Check sheet for the modelled part. Datum: model origin and axes. Units: mm. Face numbers are marked on the shaded views. A direction names the side the tool comes from. Give positions to 0.01 mm unless a question says otherwise; leave off trailing zeros. Write each loop counter-clockwise with the first axis right and the second up, starting at its lowest first coordinate (ties: lowest second). Pieces come first, ordered by that corner, then holes. Notation, with made-up numbers: M 25.5,-11.5 L 82.5,-11.5 A23 ccw 82.5,-0.5 Z; hole C 62,76 d11. An arc over 180 degrees is marked long. Use CSV: the item, a comma, the result in double quotes. Start each with the question number.
1. Cross-section at D-D, the plane y = -23.5. Enter the section's corners in (x, z).
2. Cross-section at C-C, the plane z = 43. Enter the section's corners in (x, y), and give its area (3 significant figures).
3. Depth check by flat-ended pin: P1, Ø1.4, axis at x = -41, y = -39.5, coming from the +Z side; P2, Ø1.5, axis at y = -21, z = 117, coming from the +X side; P3, Ø11, axis at x = -15.5, y = -47, coming from the -Z side; P4, Ø5, axis at x = -32, z = 81, coming from the +Y side. Enter the tip coordinate at first touch or a pass-through.
4. Scan lines: line 1 (Z direction, x = -58, y = -8.5); line 2 (X direction, y = -19, z = 56.5); line 3 (Y direction, x = -10.5, z = 86.5). Record each from-to range of solid material in increasing order.
5. Access from +Z, -Z, +X, -X, +Y, -Y to the whole of each face (thin tool, end or side, straight path). Record for the marked faces 4 and 5.
6. Cross-section at B-B, the plane x = -40. Enter the section's corners in (y, z), and give its area (3 significant figures).
7. Cross-section at A-A, the plane y = -30. Enter the section's corners in (x, z), and give its area (3 significant figures).
8. Mould release check, pull along Z, two halves, no side actions. Record for the marked faces 1, 2 and 3: +Z half, -Z half, draft (parallel to the pull), parting line (faces both ways), or undercut.
from build123d import *

# Parameters (mm, degrees)
F0_W      = 80
F0_H      = 120
F1_DEPTH  = 40
F2_T      = -1.8
F0_H_2    = 10
F3_DEPTH  = 40
F5_DEPTH  = 40
F8_DEPTH  = 5
F9_DEPTH  = 6
F10_DEPTH = 10
F12_DEPTH = 5


with BuildPart() as f1:
    # F0 (on Front) → F1 (new body)
    with BuildSketch(Plane.XZ):
        with Locations((-40, 60)):
            Rectangle(F0_W, F0_H)
    extrude(amount=F1_DEPTH)

    # F2
    f2_openings = [f1.faces().sort_by_distance(p)[0] for p in [
        (-40, 0, 60),
    ]]
    offset(amount=F2_T, openings=f2_openings)

    # F0 (on Front) → F3 (join)
    with BuildSketch(Plane.XZ):
        with Locations((-40, 125)):
            Rectangle(F0_W, F0_H_2)
    extrude(amount=F3_DEPTH)

    # F4 (on face) → F5 (cut)
    with BuildSketch(Plane.XZ):
        Polygon((-42.5, 45), (-40, 45), (-37.5, 45), (-37.5, 75), (-42.5, 75), align=None)
    extrude(amount=F5_DEPTH, mode=Mode.SUBTRACT)

    # F7 (on offset) → F8 (join)
    with BuildSketch(Plane.XY.offset(130)):
        with BuildLine():
            ThreePointArc((-50, 0), (-40, -10), (-30, 0))
            Line((-30, 0), (-40, 0))
            Line((-40, 0), (-50, 0))
        make_face()
    extrude(amount=F8_DEPTH)

    # F7 (on offset) → F9 (cut)
    with BuildSketch(Plane.XY.offset(130)):
        with BuildLine():
            ThreePointArc((-12, -20), (-14.343146, -14.343146), (-20, -12))
            ThreePointArc((-20, -12), (-28, -20), (-20, -28))
            ThreePointArc((-20, -28), (-14.343146, -25.656854), (-12, -20))
        make_face()
        with BuildLine():
            ThreePointArc((-52, -20), (-54.343146, -14.343146), (-60, -12))
            ThreePointArc((-60, -12), (-68, -20), (-60, -28))
            ThreePointArc((-60, -28), (-54.343146, -25.656854), (-52, -20))
        make_face()
    extrude(amount=-F9_DEPTH, mode=Mode.SUBTRACT)

    # F7 (on offset) → F10 (join)
    with BuildSketch(Plane.XY.offset(130)):
        with BuildLine():
            ThreePointArc((-50, -40), (-52.928932, -32.928932), (-60, -30))
            ThreePointArc((-60, -30), (-67.071068, -47.071068), (-50, -40))
        make_face()
        with BuildLine():
            ThreePointArc((-10, -40), (-12.928932, -32.928932), (-20, -30))
            ThreePointArc((-20, -30), (-27.071068, -47.071068), (-10, -40))
        make_face()
    extrude(amount=-F10_DEPTH)

    # F11 (on offset) → F12 (cut)
    with BuildSketch(Plane.XY.offset(130)):
        with BuildLine():
            ThreePointArc((-70, -40), (-60, -50), (-50, -40))
            Line((-50, -40), (-60, -40))
            Line((-60, -40), (-70, -40))
        make_face()
        with BuildLine():
            ThreePointArc((-30, -40), (-20, -50), (-10, -40))
            Line((-10, -40), (-20, -40))
            Line((-20, -40), (-30, -40))
        make_face()
    extrude(amount=-F12_DEPTH, mode=Mode.SUBTRACT)


solid = f1.part
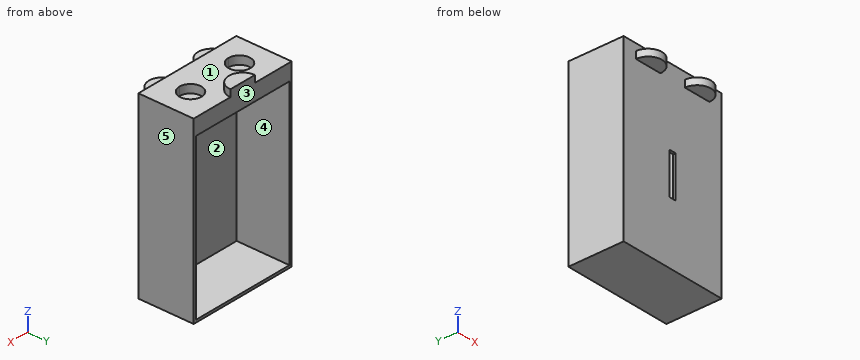
Worked answers:
1,outline,"M -80,0 L 0,0 L 0,130 L -12.81,130 L -12.81,124 L -27.19,124 L -27.19,130 L -52.81,130 L -52.81,124 L -67.19,124 L -67.19,130 L -80,130 Z; hole M -78.2,1.8 L -1.8,1.8 L -1.8,118.2 L -78.2,118.2 Z"
2,outline,"M -80,-40 L 0,-40 L 0,0 L -1.8,0 L -1.8,-38.2 L -78.2,-38.2 L -78.2,0 L -80,0 Z"
2,area,"282 mm^2"
3,P1,"stops at z = 130"
3,P2,"stops at x = 0"
3,P3,"stops at z = 120"
3,P4,"stops at y = -38.2"
4,line 1,"z = 0 to 1.8, 118.2 to 130"
4,line 2,"x = -80 to -78.2, -1.8 to 0"
4,line 3,"y = -40 to -38.2"
5,face 4,"+Y"
5,face 5,"+Z, -Z, +X, +Y, -Y"
6,outline,"M -40,0 L 0,0 L 0,1.8 L -38.2,1.8 L -38.2,45 L -40,45 Z; M -40,75 L -38.2,75 L -38.2,118.2 L 0,118.2 L 0,135 L -10,135 L -10,130 L -40,130 Z"
6,area,"750 mm^2"
7,outline,"M -80,0 L 0,0 L 0,130 L -80,130 Z; hole M -78.2,1.8 L -1.8,1.8 L -1.8,118.2 L -78.2,118.2 Z"
7,area,"1,510 mm^2"
8,face 1,"+Z half"
8,face 2,"undercut"
8,face 3,"draft"
